Here's how the part is built. I have some questions about the finished solid (model axes, mm). Coordinates: 2 decimals unless noted, no trailing zeros. Write each loop counter-clockwise with the first axis right and the second up, starting at its lowest first coordinate (ties: lowest second). Pieces come first, ordered by that corner, then holes.
from build123d import *

# Parameters (mm, degrees)
SKETCH1_R           = 2.645472677
BOSS_EXTRUDE1_DEPTH = 2.54


with BuildPart() as part:
    # Sketch1 → Boss-Extrude1 (new body)
    # profile 1 of 2: a face of its own
    with BuildSketch(Plane.XY):
        with BuildLine():
            ThreePointArc((2.715551876, 28.591516871), (0.719669389, 26.320778151), (0, 23.384474828))
            Line((0, 23.384474828), (0, 6.35))
            ThreePointArc((0, 6.35), (1.859871939, 1.859871939), (6.35, 0))
            Line((6.35, 0), (39.703606091, 0))
            Line((39.703606091, 0), (39.703606091, 27.523486691))
            ThreePointArc((39.703606091, 27.523486691), (24.126563096, 25.131896001), (9.984448124, 18.177432785))
            ThreePointArc((9.984448124, 18.177432785), (5.563703041, 18.963729745), (6.35, 23.384474828))
            ThreePointArc((6.35, 23.384474828), (22.221598132, 31.189420948), (39.703606091, 33.873486691))
            Line((39.703606091, 33.873486691), (39.703606091, 40.223486691))
            ThreePointArc((39.703606091, 40.223486691), (20.316633168, 37.246945895), (2.715551876, 28.591516871))
        make_face()
        with Locations((6.35, 6.35)):
            Circle(SKETCH1_R, mode=Mode.SUBTRACT)
    # profile 2 of 2: a face of its own
    with BuildSketch(Plane.XY):
        with BuildLine():
            ThreePointArc((76.691660306, 28.591516871), (59.090579014, 37.246945895), (39.703606091, 40.223486691))
            Line((39.703606091, 40.223486691), (39.703606091, 33.873486691))
            ThreePointArc((39.703606091, 33.873486691), (57.18561405, 31.189420948), (73.057212182, 23.384474828))
            ThreePointArc((73.057212182, 23.384474828), (73.843509142, 18.963729745), (69.422764059, 18.177432785))
            ThreePointArc((69.422764059, 18.177432785), (55.280649086, 25.131896001), (39.703606091, 27.523486691))
            Line((39.703606091, 27.523486691), (39.703606091, 0))
            Line((39.703606091, 0), (73.057212182, 0))
            ThreePointArc((73.057212182, 0), (77.547340243, 1.859871939), (79.407212182, 6.35))
            Line((79.407212182, 6.35), (79.407212182, 23.384474828))
            ThreePointArc((79.407212182, 23.384474828), (78.687542794, 26.320778151), (76.691660306, 28.591516871))
        make_face()
        with Locations((73.057212182, 6.35)):
            Circle(SKETCH1_R, mode=Mode.SUBTRACT)
    extrude(amount=-BOSS_EXTRUDE1_DEPTH)


solid = part.part
1. I want a section at C-C (y = 22). List the corners of the cut face in (x, z) for me.
2. If I drill on line 1 (Y direction, x = 6.35, z = -0.85); line 2 (Y direction, x = 45, z = -2.2); line 3 (Y direction, x = 54.5, z = -2.05), over which ranges is the centre line in solid material (lowest first)?
3. I want a section at D-D (x = 66). List the corners of the cut face in (y, z) for me.
4. For pin 1 Ø1.5 at (x, z) = (68, -0.5) entering from +Y, with a flat end and sliding along its axis, tell me the tip position at first contact or that it passes through.
5. Thinking about a two-plate mould opening in Y: for faces 1 (the face through (0.74, 26.36, -1.25)), 2 (the face through (77.498, 1.811, -1.252)), 3 (the face through (7.571, 4.003, -1.252)), which applies, pulls with the +Y half, pulls with the -Y half, needs draft (parallel to the pull), parting line crosses it, or undercut?
6. I want a section at B-B (x = 11.5). List the corners of the cut face in (y, z) for me, then the cut area to 3 significant figures.
7. I want a section at A-A (z = -0.95). List the corners of the cut face in (x, y) for me (3 decimals).
Response values:
1. outline: (0, -2.54) - (5.24, -2.54) - (5.24, 0) - (0, 0) - close; (16.4, -2.54) - (63.01, -2.54) - (63.01, 0) - (16.4, 0) - close; (74.17, -2.54) - (79.41, -2.54) - (79.41, 0) - (74.17, 0) - close
2. line 1: y = 0 to 3.7, 9 to 18.18, 23.38 to 30.95
2. line 2: y = 0 to 27.25, 33.63 to 40.01
2. line 3: y = 0 to 25.37, 31.96 to 38.51
3. outline: (0, -2.54) - (20.37, -2.54) - (20.37, 0) - (0, 0) - close; (27.6, -2.54) - (34.63, -2.54) - (34.63, 0) - (27.6, 0) - close
4. pin 1: stops at y = 34.06
5. face 1: pulls with the +Y half
5. face 2: pulls with the -Y half
5. face 3: undercut
6. outline: (0, -2.54) - (19.2, -2.54) - (19.2, 0) - (0, 0) - close; (26.59, -2.54) - (33.74, -2.54) - (33.74, 0) - (26.59, 0) - close
6. area: 66.9 mm2
7. outline: (0, 6.35) arc R6.35 ccw to (6.35, 0) - (73.057, 0) arc R6.35 ccw to (79.407, 6.35) - (79.407, 23.384) arc R6.35 ccw to (76.692, 28.592) arc R64.624 ccw to (2.716, 28.592) arc R6.35 ccw to (0, 23.384) - close; hole circle Ø5.291 at (6.35, 6.35); hole (6.35, 23.384) arc R3.175 ccw to (9.984, 18.177) arc R51.924 cw to (69.423, 18.177) arc R3.175 ccw to (73.057, 23.384) arc R58.274 ccw to start; hole circle Ø5.291 at (73.057, 6.35)
